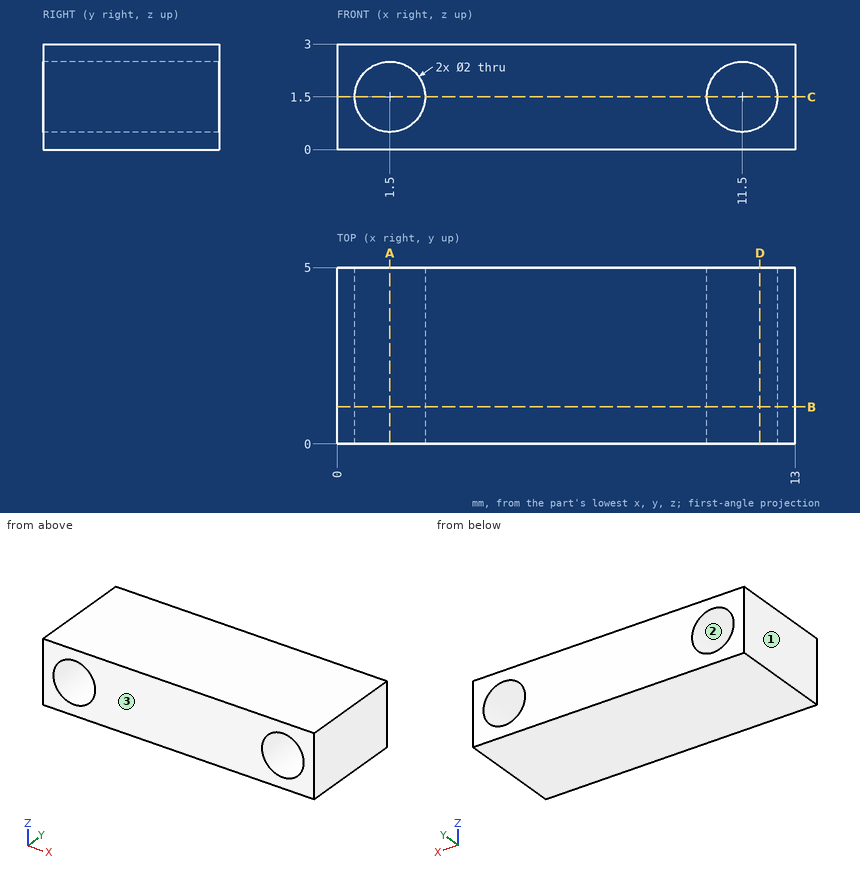
The drawing under review shows one solid part. Ordinate dimensions are in mm from its lowest x, y, z. Coordinates: 2 decimals unless noted, no trailing zeros. Write each loop counter-clockwise with the first axis right and the second up, starting at its lowest first coordinate (ties: lowest second). Pieces come first, ordered by that corner, then holes. Notation, with made-up numbers: (21, 19) -> (46, 19) arc R13 ccw to (46, 39) -> close; hole circle Ø9 at (89, 25.5). An arc over 180 degrees is marked (long way). Write each question's results on one line, items separated by ' | '. Start each with the question number.
1) Wall thickness on L1, parallel to Z at x = 11.5, y = 1.25; L2, parallel to X at y = 1.3, z = 0.6; L3, parallel to X at y = 4.45, z = 1.4: over which ranges is each line inside the solid? List them lowest first. Write a range as [from, to].
2) Consider section A-A (x = 1.5). Write out the cut boundary in (y, z).
3) Consider section C-C (z = 1.5). Write out the cut boundary in (x, y).
4) Consider section B-B (y = 1.05). Write out the cut boundary in (x, z), plus the area to 3 significant figures.
5) Consider section D-D (x = 12). Write out the cut boundary in (y, z).
6) The part is to be moulded in two halves that separate along X. For the marked faces 1, 2 and 3, say which applies: +X half, -X half, draft (parallel to the pull), parting line (faces both ways), or undercut.
Geometry says:
1) L1: [0, 0.5], [2.5, 3] | L2: [0, 1.06], [1.94, 11.06], [11.94, 13] | L3: [0, 0.51], [2.49, 10.51], [12.49, 13]
2) outline: (0, 0) -> (5, 0) -> (5, 0.5) -> (0, 0.5) -> close; (0, 2.5) -> (5, 2.5) -> (5, 3) -> (0, 3) -> close
3) outline: (0, 0) -> (0.5, 0) -> (0.5, 5) -> (0, 5) -> close; (2.5, 0) -> (10.5, 0) -> (10.5, 5) -> (2.5, 5) -> close; (12.5, 0) -> (13, 0) -> (13, 5) -> (12.5, 5) -> close
4) outline: (0, 0) -> (13, 0) -> (13, 3) -> (0, 3) -> close; hole circle Ø2 at (1.5, 1.5); hole circle Ø2 at (11.5, 1.5) | area: 32.7 mm^2
5) outline: (0, 0) -> (5, 0) -> (5, 0.63) -> (0, 0.63) -> close; (0, 2.37) -> (5, 2.37) -> (5, 3) -> (0, 3) -> close
6) face 1: -X half | face 2: undercut | face 3: draft
